Source: CAD feature listing. Evaluate the final solid. Frame: model axes, mm. A direction names the side the tool comes from. Round coordinates to 2 decimals unless told otherwise and drop trailing zeros. Order: outer loops, then holes, each group sorted by start corner. A loop starts at its lowest first (then second) coordinate and runs counter-clockwise, first axis right, second up. Notation, with made-up numbers: M 27.5,61 L 45.5,61 A21 ccw 45.5,92 Z; hole C 71.5,-34.5 d9. An arc over 180 degrees is marked long. Use CSV: the item, a comma, the result in double quotes. Start each with the question number.
```python
from build123d import *

# Parameters (mm, degrees)
SALIENTE_EXTRUIR1_DEPTH      = 5
SALIENTE_EXTRUIR1_DEPTH_BACK = 5
CROQUIS6_3_R                 = 10
CROQUIS6_3_R_2               = 5
SALIENTE_EXTRUIR2_DEPTH      = 7
SALIENTE_EXTRUIR2_DEPTH_BACK = 7


with BuildPart() as part:
    # Croquis6 → Saliente-Extruir1 (new body, two sides)
    with BuildSketch(Plane(origin=(0, 0, 0), x_dir=(1, 0, 0), z_dir=(0, 1, 0))) as saliente_extruir1_sk:
        with BuildLine():
            Line((-7.5, 23.848480035), (-53, 9.539392014))
            ThreePointArc((-53, 9.539392014), (-44.083920217, 8.062257748), (-40, 0))
            ThreePointArc((-40, 0), (-44.083920217, -8.062257748), (-53, -9.539392014))
            Line((-53, -9.539392014), (-7.5, -23.848480035))
            ThreePointArc((-7.5, -23.848480035), (0, -25), (7.5, -23.848480035))
            Line((7.5, -23.848480035), (53, -9.539392014))
            ThreePointArc((53, -9.539392014), (40, 0), (53, 9.539392014))
            Line((53, 9.539392014), (7.5, 23.848480035))
            ThreePointArc((7.5, 23.848480035), (0, 25), (-7.5, 23.848480035))
        make_face()
        with BuildLine():
            Line((12, -8), (-12, -8))
            ThreePointArc((-12, -8), (-20, 0), (-12, 8))
            Line((-12, 8), (12, 8))
            ThreePointArc((12, 8), (20, 0), (12, -8))
        make_face(mode=Mode.SUBTRACT)
    extrude(amount=SALIENTE_EXTRUIR1_DEPTH)
    extrude(saliente_extruir1_sk.sketch, amount=-SALIENTE_EXTRUIR1_DEPTH_BACK)

    # Croquis6_3 → Saliente-Extruir2 (add, two sides)
    with BuildSketch(Plane(origin=(0, 0, 0), x_dir=(1, 0, 0), z_dir=(0, 1, 0))) as saliente_extruir2_sk:
        with Locations((50, 0)):
            Circle(CROQUIS6_3_R)
        with Locations((50, 0)):
            Circle(CROQUIS6_3_R_2, mode=Mode.SUBTRACT)
        with Locations((-50, 0)):
            Circle(CROQUIS6_3_R)
        with Locations((-50, 0)):
            Circle(CROQUIS6_3_R_2, mode=Mode.SUBTRACT)
    extrude(amount=SALIENTE_EXTRUIR2_DEPTH)
    extrude(saliente_extruir2_sk.sketch, amount=-SALIENTE_EXTRUIR2_DEPTH_BACK)


solid = part.part
```
(1) Section A-A on y = 1.5. Return loops of the section in (x, z).
(2) Section B-B on z = 0. Return loops of the section in (x, y), plus the area to 3 significant figures.
(3) Line query: line 1 along X through (y, z) = (-5.25, 0); line 2 along X through (y, z) = (4, 0); line 3 along Y through (x, z) = (12, 16). Output: solid intervals per line, ascending.
(4) Reachability of faces 5 (the face through (45, 7, 2)), 6 (the face through (20, 0, 0)) from +Z, -Z, +X, -X, +Y, -Y: full face, straight path, thin tool, end or side. Return the list, or none.
(5) Section C-C on x = 18. Return loops of the section in (y, z).
(6) Contact query for flat-ended pins moving along their axis: P1, Ø1, axis at x = 23.5, z = 4.5, coming from the -Y side; P2, Ø25, axis at x = 5, z = -1, coming from the +Y side; P3, Ø3, axis at x = -22, y = -0.5, coming from the +Z side; P4, Ø8, axis at x = 50, z = 0, coming from the +Y side. Output: stop coordinate, or through.
(7) Section D-D on x = 50. Return loops of the section in (y, z).
(8) Draft query along X for faces 1 (the face through (-55, 7, 2)), 2 (the face through (0, 0, 25)), 3 (the face through (-20, 0, 0)), 4 (the face through (0, 0, 8)). Return one class per face: pulls with the +X half, pulls with the -X half, needs draft (parallel to the pull), parting line crosses it, or undercut.
Results below:
1,outline,"M -53,-9.54 L -7.5,-23.85 A25 ccw 7.5,-23.85 L 53,-9.54 A10 ccw 53,9.54 L 7.5,23.85 A25 ccw -7.5,23.85 L -53,9.54 A10 ccw Z; hole C -50,0 d10; hole M -12,-8 L 12,-8 A8 ccw 12,8 L -12,8 A8 ccw Z; hole C 50,0 d10"
2,outline,"M -60,-7 L -55,-7 L -55,7 L -60,7 Z; M -45,-7 L -40,-7 L -40,-5 L -20,-5 L -20,5 L -40,5 L -40,7 L -45,7 Z; M 20,-5 L 40,-5 L 40,-7 L 45,-7 L 45,7 L 40,7 L 40,5 L 20,5 Z; M 55,-7 L 60,-7 L 60,7 L 55,7 Z"
2,area,"680 mm2"
3,line 1,"x = -60 to -55, -45 to -40, 40 to 45, 55 to 60"
3,line 2,"x = -60 to -55, -45 to -20, 20 to 45, 55 to 60"
3,line 3,"y = -5 to 5"
4,face 5,"+Z, -Z, +X, -X, +Y"
4,face 6,"+Y, -Y"
5,outline,"M -5,-20.55 L 5,-20.55 L 5,-5.29 L -5,-5.29 Z; M -5,5.29 L 5,5.29 L 5,20.55 L -5,20.55 Z"
6,P1,"stops at y = -5"
6,P2,"stops at y = 5"
6,P3,"stops at z = 19.76"
6,P4,"passes through"
7,outline,"M -7,-10 L -5,-10 L -5,-10.48 L 5,-10.48 L 5,-10 L 7,-10 L 7,-5 L -7,-5 Z; M -7,5 L 7,5 L 7,10 L 5,10 L 5,10.48 L -5,10.48 L -5,10 L -7,10 Z"
8,face 1,"needs draft"
8,face 2,"parting line crosses it"
8,face 3,"undercut"
8,face 4,"undercut"
